CAD build for the part. Positions are in the model's coordinates, mm. A direction names the side the tool comes from. Coordinates: 2 decimals unless noted, no trailing zeros. Loops run counter-clockwise (first coordinate to the right, second up) from the corner with the lowest first, then second, coordinate; pieces in that order, holes last. Notation, with made-up numbers: (-38.5, 86.5) -> (2.5, 86.5) arc R23 ccw to (2.5, 102.5) -> close; hole circle Ø7 at (-10, 25.5). An arc over 180 degrees is marked (long way). Answer as a JSON object with one key per item and string values. Group by question number.
from build123d import *

# Parameters (mm, degrees)
FILLET1_R = 0.2


with BuildPart() as part:
    # Sketch 1 → Body (revolve)
    with BuildSketch(Plane.XY, mode=Mode.PRIVATE) as body_sk:
        Polygon((1, 7.5), (1, 2.611783382), (1.086628376, 2.5), (1, 2.388216618), (1, 1.1), (14, 1.1), (14, 2.411783382), (13.9, 2.511783382), (14, 2.611783382), (14, 7.5), (13.04, 7.5), (13.04, 4.5), (1.96, 4.5), (1.96, 7.5), align=None)
    revolve(body_sk.sketch.rotate(Axis((1, -1.5, 0), (1, 0, 0)), 90), axis=Axis((1, -1.5, 0), (1, 0, 0)))

    # Fillet1
    fillet1_edges = [part.edges().sort_by_distance(p)[0] for p in [
        (14, -1.5, -2.6),
        (1, -1.5, -2.6),
    ]]
    fillet(fillet1_edges, radius=FILLET1_R)


solid = part.part
Item 1: Flat gauge pins, fed straight in: P1, Ø3, axis at x = 3, y = -1.5, coming from the +Z side; P2, Ø2, axis at x = 12, z = 3.5, coming from the +Y side; P3, Ø2, axis at x = 3.5, y = 0.5, coming from the +Z side; P4, Ø1.5, axis at x = 12, z = 2.5, coming from the -Y side. Where does each tip first touch, or does it go through?
Item 2: 3-axis set-ups, long thin cutter, end or side, ignore diameter. For faces 4 (the flat face through (14, 0, -4)), 5 (the flat face through (1.96, 4.4, -1.9)): which of +Z, -Z, +X, -X, +Y, -Y reach the whole face in a straight line?
Item 3: Pull direction Y, two halves, no side cores. Call faces 1 (the cylindrical face through (13.513, 7.286, -1.951)), 2 (the cylindrical face through (7.59, 1.04, -0.56)), 3 (the flat face through (1, 0, 4)): +Y half, -Y half, draft (parallel to the pull), parting line (faces both ways), or undercut.
Item 4: Band-saw the part on C-C, the plane x = 7.25. List the corners of the cut face in (y, z), and give its area (3 significant figures).
Item 5: Band-saw the part on D-D, the plane y = 3.75. List the corners of the cut face in (x, z).
Item 6: Drill centre lines: L1, parallel to X at y = 5.25, z = -3.5; L2, parallel to Y at x = 8.5, z = 0; L3, parallel to Y at x = 8.75, z = 1.75. Where is each one in solid material? Low to high.
Reply:
{
 "1": {"P1": "z = 9", "P2": "y = 3.95", "P3": "z = 5.92", "P4": "y = -7.24"},
 "2": {"face 4": "+Z, -Z, +X, +Y, -Y", "face 5": "none"},
 "3": {"face 1": "parting line", "face 2": "undercut", "face 3": "draft"},
 "4": {"outline": "circle Ø12 at (-1.5, 0); hole circle Ø5.2 at (-1.5, 0)", "area": "91.9 mm²"},
 "5": {"outline": "(1, -7.31) -> (1.96, -7.31) -> (1.96, -2.9) -> (13.04, -2.9) -> (13.04, -7.31) -> (14, -7.31) -> (14, 7.31) -> (13.04, 7.31) -> (13.04, 2.9) -> (1.96, 2.9) -> (1.96, 7.31) -> (1, 7.31) -> close"},
 "6": {"L1": "1 to 1.96, 13.04 to 14", "L2": "-7.5 to -4.1, 1.1 to 4.5", "L3": "-7.24 to -3.42, 0.42 to 4.24"}
}
